For this review, take the finished solid that the model builds, in its own axes (mm). Give positions to 0.01 mm unless a question says otherwise; leave off trailing zeros. Write each loop counter-clockwise with the first axis right and the second up, starting at its lowest first coordinate (ties: lowest second). Pieces come first, ordered by that corner, then holes. Notation, with made-up numbers: (53.25, -20.5) -> (75.25, -20.5) arc R8 cw to (75.25, -15.5) -> close; hole circle Ø7 at (39.5, -40). An arc over 180 degrees is marked (long way). Write item = value, one per line.
```python
from build123d import *

# Parameters (mm, degrees)
CYLINDER001_R     = 600
CYLINDER001_DEPTH = 1200
CYLINDER_R        = 600
CYLINDER_DEPTH    = 1200


with BuildPart() as cylinder001:
    # Cylinder001 → Cylinder001 (new body)
    with BuildSketch(Plane.XY.offset(-654)):
        Circle(CYLINDER001_R)
    extrude(amount=CYLINDER001_DEPTH)


with BuildPart() as cut001:
    # Sphere001 → Sphere001 (revolve)
    with BuildSketch(Plane.XZ):
        with BuildLine():
            ThreePointArc((0, -600), (600, 0), (0, 600))
            Line((0, 600), (0, -600))
        make_face()
    revolve(axis=Axis((0, 0, 0), (0, 0, 1)))

    # Cut001: cut Cylinder001
    add(cylinder001.part, mode=Mode.SUBTRACT)


with BuildPart() as cut001_1:
    # Cut001 placement: moved
    add(cut001.part.moved(Location((0, 0, -3))))


with BuildPart() as cylinder:
    # Cylinder → Cylinder (new body)
    with BuildSketch(Plane.XY.offset(-654)):
        Circle(CYLINDER_R)
    extrude(amount=CYLINDER_DEPTH)


with BuildPart() as cut002:
    # Sphere → Sphere (revolve)
    with BuildSketch(Plane.XZ):
        with BuildLine():
            ThreePointArc((0, -600), (600, 0), (0, 600))
            Line((0, 600), (0, -600))
        make_face()
    revolve(axis=Axis((0, 0, 0), (0, 0, 1)))

    # Cut: cut Cylinder
    add(cylinder.part, mode=Mode.SUBTRACT)

    # Cut002: cut Cut001
    add(cut001_1.part, mode=Mode.SUBTRACT)


solid = cut002.part
```
(1) Take a section at B-B (x = 145). Write out the cut boundary in (y, z), plus the area to 3 significant figures.
Answers below:
outline = (-202.14, 546) -> (-193.84, 546) arc R582.22 cw to (193.84, 546) -> (202.14, 546) arc R582.22 ccw to start
area = 1,190 mm^2
(2) To check wall thickness, follow probe 1 along Z at (x, y) = (-18.5, 22); probe 2 along Z at (x, y) = (112, 87). State the ranges of each line that lie inside material, in increasing order.
Answers below:
probe_1 = 596.31 to 599.31
probe_2 = 580 to 583
(3) Take a section at A-A (z = 565). Write out the cut boundary in (x, y), plus the area to 3 significant figures.
Answers below:
outline = circle Ø403.86 at (0, 0); hole circle Ø386.66 at (0, 0)
area = 10,700 mm^2
(4) For pin 1 (2 mm diameter, centred on x = -92.5, y = 1, fed in from +Z); pin 2 (10 mm diameter, centred on y = -75.5, z = 552, fed in from -X); pin 3 (3 mm diameter, centred on x = 85, y = 137.5, fed in from -Z), all flat-tipped, find the tip position at first contact; note any pin that passes through.
Answers below:
pin_1 = 592.98
pin_2 = -234.82
pin_3 = 574.39
(5) Take a section at C-C (y = -102.5). Write out the cut boundary in (x, z).
Answers below:
outline = (-226.67, 546) -> (-219.3, 546) arc R591.18 cw to (219.3, 546) -> (226.67, 546) arc R591.18 ccw to start
